Autodesk Inventor part; units mm, degrees
ref_plane "YZ Plane" through (0, 0, 0) normal (1, 0, 0) x (0, 1, 0)
ref_plane "XZ Plane" through (0, 0, 0) normal (0, 1, 0) x (-1, 0, 0)
ref_plane "XY Plane" through (0, 0, 0) normal (0, 0, 1) x (1, 0, 0)
sketch "Skizze2" plane through (0, 0, 0) normal (0, 1, 0) x (-1, 0, 0)
  arc A0 (-4.0562, -0.75) -> (-4.0562, 0.75) centre (0, 0) ccw
  line L0 (8.75, -7.8806) -> (-8.75, -7.8806)
  line L1 (-8.75, -7.8806) -> (-8.75, 5.925)
  line L2 (-8.75, 5.925) -> (8.75, 5.925)
  line L3 (8.75, 5.925) -> (8.75, -7.8806)
  line L4 (8.75, -4.6225) -> (8.75, -1.5)
  arc A1 (8.75, 1.925) -> (8.75, -1.925) centre (7.9934, 0) ccw
  line L5 (8.75, -7.8806) -> (-8.75, -7.8806)
  line L6 (-8.75, -7.8806) -> (-8.75, -5.4806)
  line L7 (-8.75, -5.4806) -> (8.75, -5.4806)
  line L8 (8.75, -5.4806) -> (8.75, -7.8806)
  line L9 (2.25, -5.4806) -> (2.25, -3.4573)
  line L10 (-2.25, -5.4806) -> (-2.25, -3.4573)
  arc A2 (-2.25, -3.4573) -> (2.25, -3.4573) centre (0, 0) ccw
  line L11 (2.25, -5.4806) -> (-2.25, -5.4806)
  line L12 (-4.0562, -0.75) -> (-8.75, -0.75)
  line L13 (-4.0562, 0.75) -> (-8.75, 0.75)
  arc A3 (8.75, 1.925) -> (4.75, 5.925) centre (4.75, 1.925) ccw
  arc A4 (-4.75, 5.925) -> (-8.75, 1.925) centre (-4.75, 1.925) ccw
  line L14 (0, -10.8073) -> (0, 9.6802) construction
  line L15 (8.75, 0) -> (-8.75, 0) construction
  point P0 (5.25, -5.4806)
  point P1 (-5.25, -5.4806)
  dimension "d0" = 8.25
  dimension "d2" = 17.5
  dimension "d4" = 1.8
  dimension "d7" = 2.4
  dimension "d8" = 1.5
  dimension "d10" = 4
  dimension "d11" = 10.5
  dimension "d12" = 3
  dimension "d38" = 1.8
  dimension "d39" = 1.3556
extrude "Extrusion2" add sketch "Skizze2" against normal blind 14.5 contours A0 L10 L7 L1 L12 | A0 L9 L7 L10 | A0 L13 L1 A4 L2 A3 A1 L3 L7 L9 | L7 L3 L0 L1
extrude "Extrusion3" add sketch "Skizze2" along normal blind 6 contours A0 L9 L7 L10 | L7 L3 L0 L1
sketch "Skizze3" plane through (-8.75, 0, -5.4806) normal (0, 0, 1) x (1, 0, 0)
  line L0 (0, -14.5) -> (0, 0)
  line L1 (0, 0) -> (0, 6)
  line L2 (0, 6) -> (6.5, 6)
  line L3 (6.5, 6) -> (11, 6)
  line L4 (11, 6) -> (11, 0)
  line L5 (11, 0) -> (17.5, 0)
  line L6 (17.5, 6) -> (17.5, 0)
  line L7 (11, 6) -> (17.5, 6)
  line L8 (17.5, -14.5) -> (0, -14.5)
  line L9 (17.5, 0) -> (17.5, -14.5)
  line L10 (0, 0) -> (6.5, 0)
  line L11 (6.5, 0) -> (6.5, 6)
  line L12 (3.5, 0) -> (3.5, 6) construction
  line L13 (0, 6) -> (6.5, 6)
  line L14 (14, 0) -> (14, 6) construction
  line L15 (11, 6) -> (17.5, 6)
  point P0 (8.75, 0)
  point P1 (3.5, 3)
  point P2 (14, 3)
hole "Bohrung1" at (-5.25, 3, -5.4806) at (5.25, 3, -5.4806) direction (0, 0, -1) diameter 3.4 end through all
fillet "Rundung1" radius 2 2 edges at (-8.75, 6, -6.6806) (8.75, 6, -6.6806)
sketch "Skizze4" plane through (-4.75, 0, 5.925) normal (0, 0, 1) x (1, 0, 0)
  line L0 (8.8062, 0) -> (13.5, 0)
  line L1 (8.8062, 0) -> (8.8062, -14.5)
  line L2 (13.5, -14.5) -> (8.8062, -14.5)
  line L3 (13.5, 0) -> (13.5, -14.5)
  line L4 (13.5, 0) -> (9.5, 0)
  line L5 (10.5, -14.5) -> (10.5, 0) construction
  point P0 (4.75, 0)
  point P1 (10.5, -7.25)
  dimension "d30" = 3
hole "Bohrung2" at (5.75, -7.25, 5.925) direction (0, 0, -1) diameter 3.2 end through all counterbore diameter 6 counterbore depth 2
sketch "Skizze5" plane through (8.75, -14.5, -7.8806) normal (0, 0, -1) x (-1, 0, 0)
  circle A0 centre (3, 7.25) radius 1.6
  point P0 (8.75, 14.5)
hole "Bohrung3" at (5.75, -7.25, -7.8806) direction (0, 0, 1) diameter 4.5 depth 5
properties part number "Vinda_Mount_v2" material "Stahl"
Check sheet for the modelled part. Datum: model origin and axes. Units: mm. A direction names the side the tool comes from. Give positions to 0.01 mm unless a question says otherwise; leave off trailing zeros. Loops run counter-clockwise (first coordinate to the right, second up) from the corner with the lowest first, then second, coordinate; pieces in that order, holes last. Notation, with made-up numbers: (43.5, -38) - (91.5, -38) arc R25 ccw to (91.5, -23) - close; hole circle Ø2 at (68, -39.75). An arc over 180 degrees is marked (long way). One line per question, with ' | ' between items. Start each with the question number.
1. Material ranges on line 1 along Z through (x, y) = (0, -5.25) (3 decimals); line 2 along X through (y, z) = (-7.75, 1.25); line 3 along X through (y, z) = (-4, 0), recorded low to high. Write a range as [from, to].
2. Cross-section at C-C, the plane x = -2.5. Enter the section's corners in (y, z) (3 decimals), plus the area to 3 significant figures.
3. Gauge pin test, flat ends, axial feed: pin 1 Ø1.8 at (x, y) = (-5.5, 2.5) entering from +Z; pin 2 Ø1.3 at (x, y) = (6.5, -8) entering from -Z; pin 3 Ø3.5 at (x, z) = (-2.5, 2.5) entering from +Y; pin 4 Ø5 at (x, y) = (5.75, -7.25) entering from +Z (3 decimals). Record the tip position at first contact, or that the pin passes through.
4. Draft check along X on faces 4 (the flat face through (2, -14.5, -4)), 5 (the cylindrical face through (8.356, -7.148, 3.655)), 6 (the cylindrical face through (-5.926, -7.148, 0.056)). Enter one of: released by +X, released by -X, zero draft, split by the parting line, or undercut.
5. Cross-section at D-D, the plane z = 2.5. Enter the section's corners in (x, y).
6. Set-up check for faces 1 (the flat face through (4, -7, -2.881)), 2 (the flat face through (6, 0, -3)), 3 (the flat face through (8, -7, 0.75)): record each of +Z, -Z, +X, -X, +Y, -Y from which the full face is reachable in a straight line by a thin tool's end or side.
7. Cross-section at A-A, the plane z = -4.5. Enter the section's corners in (x, y), plus the area to 3 significant figures.
8. Cross-section at B-B, the plane y = -7.25. Enter the section's corners in (x, z) (3 decimals).
Check result:
1) line 1: z = [-7.881, -4.125], [4.125, 5.925] | line 2: x = [-6.35, -3.93], [3.93, 4.23], [7.27, 8.75] | line 3: x = [-5.93, -4.12]
2) outline: (-14.5, -7.881) - (6, -7.881) - (6, -5.481) - (0, -5.481) - (0, -3.281) - (-14.5, -3.281) - close; (-14.5, 3.281) - (0, 3.281) - (0, 5.925) - (-14.5, 5.925) - close | area: 119 mm2
3) pin 1: passes through | pin 2: stops at z = -2.88 | pin 3: stops at y = 0 | pin 4: stops at z = 3.925
4) face 4: zero draft | face 5: released by +X | face 6: undercut
5) outline: (-8.71, -14.5) - (-3.28, -14.5) - (-3.28, 0) - (-8.71, 0) - close; (3.28, -14.5) - (8.71, -14.5) - (8.71, 0) - (3.28, 0) - close; hole circle Ø3.2 at (5.75, -7.25)
6) face 1: -Z | face 2: +Z, +X, +Y | face 3: +X, +Y, -Y
7) outline: (-8.75, -14.5) - (8.75, -14.5) - (8.75, 0) - (2.25, 0) - (2.25, 6) - (-2.25, 6) - (-2.25, 0) - (-8.75, 0) - close; hole circle Ø4.5 at (5.75, -7.25) | area: 265 mm2
8) outline: (-8.75, -7.881) - (3.5, -7.881) - (3.5, -2.881) - (4.15, -2.881) - (4.15, -0.75) - (4.056, -0.75) arc R4.125 cw (long way) to (4.056, 0.75) - (4.15, 0.75) - (4.15, 3.925) - (2.75, 3.925) - (2.75, 5.925) - (-4.75, 5.925) arc R4 ccw to (-8.75, 1.925) arc R2.068 cw (long way) to (-8.75, -1.925) - close; (7.35, -2.881) - (8, -2.881) - (8, -7.881) - (8.75, -7.881) - (8.75, -0.75) - (7.35, -0.75) - close; (7.35, 0.75) - (8.75, 0.75) - (8.75, 1.925) arc R4 ccw to (8.214, 3.925) - (7.35, 3.925) - close
